```python
from build123d import *

# Parameters (mm, degrees)
SKETCH1_R                  = 13.5
BOSS_EXTRUDE1_DEPTH        = 3
CAVITY26_OUTLINE_R         = 1.85
CAVITY26_OUTLINE_R_2       = 1.7
CAVITY26_DEPTH             = 1.5
F_24_0_24_DIAMETER_HOLE1_D = 3.7
BOSS_EXTRUDE2_START        = -3
SKETCH6_R                  = 13.5
BOSS_EXTRUDE2_DEPTH        = 3
F_24_0_24_DIAMETER_HOLE2_D = 5.5
SKETCH14_W                 = 5.92
SKETCH14_H                 = 13
BOSS_EXTRUDE6_DEPTH        = 9.45
SKETCH13_R                 = 4
BOSS_EXTRUDE7_DEPTH        = 6.45
BOSS_EXTRUDE8_DEPTH        = 6.45
F_24_0_24_DIAMETER_HOLE3_D = 3.7
CUT_EXTRUDE3_DEPTH         = 9.06
SKETCH19_R                 = 2.55
CUT_EXTRUDE4_DEPTH         = 1.8
CUT_EXTRUDE5_START         = -11.2
SKETCH23_R                 = 4.233528458
CUT_EXTRUDE5_DEPTH         = 2.14
SKETCH24_W                 = 2.756109072
SKETCH24_H                 = 9.9
CUT_EXTRUDE6_DEPTH         = 10
CAVITY27_DEPTH             = 1.5
CAVITY27_START             = -6.45
CAVITY27_2_OUTLINE_R       = 3.15
CAVITY27_2_OUTLINE_R_2     = 1.85
CAVITY27_2_DEPTH           = 1.8
BOSS_EXTRUDE9_START        = 1.8
SKETCH25_R                 = 6.6
SKETCH25_R_2               = 1.85
BOSS_EXTRUDE9_DEPTH        = 1.8
SKETCH26_R                 = 4.5
CUT_EXTRUDE7_DEPTH         = 3
SKETCH27_R                 = 1.85
BOSS_EXTRUDE10_DEPTH       = 3
CUT_EXTRUDE8_START         = -1.5
CUT_EXTRUDE8_DEPTH         = 1.5
CUT_EXTRUDE9_DEPTH         = 15
F_24_0_24_DIAMETER_HOLE4_D = 3.4


# Read off the part's stored shape, not the designer's step: Cavity26, Cavity27
with BuildPart() as part:
    # Sketch1 → Boss-Extrude1 (new body)
    with BuildSketch(Plane(origin=(0, 0, 0), x_dir=(1, 0, 0), z_dir=(0, 1, 0))):
        with BuildLine():
            Line((39.88, -46.3), (44.18, -42))
            Line((44.18, -42), (44.18, 0))
            Line((44.18, 0), (7, 0))
            ThreePointArc((7, 0), (2.050252532, -2.050252532), (0, -7))
            Line((0, -7), (0, -46.3))
            Line((0, -46.3), (39.88, -46.3))
        make_face()
        with Locations(Location((23.07, -25.54, 0), (0, 0, 270))):
            Circle(SKETCH1_R, mode=Mode.SUBTRACT)
    extrude(amount=BOSS_EXTRUDE1_DEPTH)

    # Cavity26 outline → Cavity26 (cut)
    # profile 1 of 2: a face of its own
    with BuildSketch(Plane(origin=(0, 0, 0), x_dir=(1, 0, 0), z_dir=(0, 1, 0))):
        with BuildLine():
            Line((40.98, -20.5), (35.593913126, -20.5))
            ThreePointArc((35.593913126, -20.5), (36.300391291, -22.855461624), (36.567866498, -25.3))
            Line((36.567866498, -25.3), (40.93, -25.3))
            Line((40.93, -25.3), (40.93, -37.4))
            Line((40.93, -37.4), (37.464525778, -37.4))
            ThreePointArc((37.464525778, -37.4), (35.919832787, -38.039832787), (35.28, -39.584525778))
            Line((35.28, -39.584525778), (35.28, -43.05))
            Line((35.28, -43.05), (12.18, -43.05))
            Line((12.18, -43.05), (12.18, -44.675))
            Line((12.18, -44.675), (39.2422583, -44.675))
            Line((39.2422583, -44.675), (42.58, -41.3372583))
            Line((42.58, -41.3372583), (42.58, -22.55))
            Line((42.58, -22.55), (40.98, -22.55))
            Line((40.98, -22.55), (40.98, -20.5))
        make_face()
        with Locations((38.63, -40.75)):
            Circle(CAVITY26_OUTLINE_R, mode=Mode.SUBTRACT)
    # profile 2 of 2: a face of its own
    with BuildSketch(Plane(origin=(0, 0, 0), x_dir=(1, 0, 0), z_dir=(0, 1, 0))):
        with BuildLine():
            Line((40.98, -6.35), (42.58, -6.35))
            Line((42.58, -6.35), (42.58, -1.6))
            Line((42.58, -1.6), (28.18, -1.6))
            Line((28.18, -1.6), (28.18, -10.6))
            Line((28.18, -10.6), (29.56, -10.6))
            Line((29.56, -10.6), (29.56, -8.2))
            Line((29.56, -8.2), (31.16, -8.2))
            Line((31.16, -8.2), (31.16, -6.35))
            Line((31.16, -6.35), (35.06, -6.35))
            Line((35.06, -6.35), (35.06, -8.4))
            Line((35.06, -8.4), (36.21908731, -8.4))
            ThreePointArc((36.21908731, -8.4), (38.578420387, -7.150450959), (40.98, -8.31674455))
            Line((40.98, -8.31674455), (40.98, -6.35))
        make_face()
        with Locations((38.08, -3.8)):
            Circle(CAVITY26_OUTLINE_R_2, mode=Mode.SUBTRACT)
    extrude(amount=CAVITY26_DEPTH, mode=Mode.SUBTRACT)

    # Ø24.0 (24) Diameter Hole1 (through all)
    with Locations(Plane(origin=(0, 3, 0), x_dir=(1, 0, 0), z_dir=(0, 1, 0))):
        with Locations((38.63, -10.1), (38.63, -40.75), (7.73, -40.75), (7.73, -10.02)):
            Hole(F_24_0_24_DIAMETER_HOLE1_D / 2)

    # Sketch6 → Boss-Extrude2 (add)
    with BuildSketch(Plane(origin=(0, 3, 0), x_dir=(1, 0, 0), z_dir=(0, 1, 0)).offset(BOSS_EXTRUDE2_START)):
        with Locations((23.07, -25.54)):
            Circle(SKETCH6_R)
    extrude(amount=BOSS_EXTRUDE2_DEPTH)

    # Ø24.0 (24) Diameter Hole2 (through all)
    with Locations(Plane(origin=(0, 3, 0), x_dir=(1, 0, 0), z_dir=(0, 1, 0))):
        with Locations((23.07, -25.54)):
            Hole(F_24_0_24_DIAMETER_HOLE2_D / 2)

    # Sketch14 → Boss-Extrude6 (add)
    with BuildSketch(Plane(origin=(0, 3, 0), x_dir=(1, 0, 0), z_dir=(0, 1, 0))):
        with Locations((-2.96, -39.8)):
            Rectangle(SKETCH14_W, SKETCH14_H)
    extrude(amount=-BOSS_EXTRUDE6_DEPTH)

    # Sketch13 → Boss-Extrude7 (add)
    with BuildSketch(Plane(origin=(0, 0, 0), x_dir=(-1, 0, 0), z_dir=(0, -1, 0))):
        with Locations(Location((-7.73, -40.75, 0), (0, 0, 270))):
            Circle(SKETCH13_R)
    extrude(amount=BOSS_EXTRUDE7_DEPTH)

    # Sketch15 → Boss-Extrude8 (add)
    with BuildSketch(Plane(origin=(0, 0, 0), x_dir=(-1, 0, 0), z_dir=(0, -1, 0))):
        with BuildLine():
            Line((-11.002613634, -43.05), (-12.18, -43.05))
            Line((-12.18, -43.05), (-12.18, -44.675))
            Line((-12.18, -44.675), (-12.18, -46.3))
            Line((-12.18, -46.3), (0, -46.3))
            Line((0, -46.3), (0, -33.3))
            Line((0, -33.3), (-6.09, -33.3))
            Line((-6.09, -33.3), (-6.09, -37.101657911))
            ThreePointArc((-6.09, -37.101657911), (-4.371428875, -38.577443902), (-3.73, -40.75))
            ThreePointArc((-3.73, -40.75), (-6.523860401, -44.563820561), (-11.002613634, -43.05))
        make_face()
    extrude(amount=BOSS_EXTRUDE8_DEPTH)

    # Ø24.0 (24) Diameter Hole3 (through all)
    with Locations(Plane(origin=(0, 3, 0), x_dir=(1, 0, 0), z_dir=(0, 1, 0))):
        with Locations((7.73, -40.75)):
            Hole(F_24_0_24_DIAMETER_HOLE3_D / 2)

    # Sketch18 → Cut-Extrude3 (cut)
    with BuildSketch(Plane(origin=(0, 0, 33.3), x_dir=(-1, 0, 0), z_dir=(0, 0, -1))):
        Polygon((-0.43, -11.856921938), (3.17, -9.778460969), (3.17, -5.621539031), (-0.43, -3.543078062), (-4.03, -5.621539031), (-4.03, -9.778460969), align=None)
    extrude(amount=-CUT_EXTRUDE3_DEPTH, mode=Mode.SUBTRACT)

    # Sketch19 → Cut-Extrude4 (cut)
    with BuildSketch(Plane.XY.offset(46.3)):
        with Locations((0.43, -7.7)):
            Circle(SKETCH19_R)
    extrude(amount=-CUT_EXTRUDE4_DEPTH, mode=Mode.SUBTRACT)

    # Sketch23 → Cut-Extrude5 (cut)
    with BuildSketch(Plane(origin=(0, 0, 33.3), x_dir=(-1, 0, 0), z_dir=(0, 0, -1)).offset(CUT_EXTRUDE5_START)):
        with Locations((-0.43, -7.7)):
            Circle(SKETCH23_R)
    extrude(amount=CUT_EXTRUDE5_DEPTH, mode=Mode.SUBTRACT)

    # Sketch24 → Cut-Extrude6 (cut)
    with BuildSketch(Plane(origin=(0, 3, 0), x_dir=(1, 0, 0), z_dir=(0, 1, 0))):
        with Locations((-1.378054536, -39.55)):
            Rectangle(SKETCH24_W, SKETCH24_H)
    extrude(amount=-CUT_EXTRUDE6_DEPTH, mode=Mode.SUBTRACT)

    # Cavity27 outline → Cavity27 (cut)
    with BuildSketch(Plane(origin=(0, 0, 0), x_dir=(1, 0, 0), z_dir=(0, 1, 0))):
        with BuildLine():
            ThreePointArc((28.18, -21.3), (29.351572875, -24.128427125), (32.18, -25.3))
            Line((32.18, -25.3), (36.567866498, -25.3))
            ThreePointArc((36.567866498, -25.3), (36.300391291, -22.855461624), (35.593913126, -20.5))
            Line((35.593913126, -20.5), (35.06, -20.5))
            Line((35.06, -20.5), (35.06, -22.55))
            Line((35.06, -22.55), (31.16, -22.55))
            Line((31.16, -22.55), (31.16, -20.7))
            Line((31.16, -20.7), (29.56, -20.7))
            Line((29.56, -20.7), (29.56, -18.3))
            Line((29.56, -18.3), (28.18, -18.3))
            Line((28.18, -18.3), (28.18, -21.3))
        make_face()
    extrude(amount=CAVITY27_DEPTH, mode=Mode.SUBTRACT)

    # Cavity27 2 outline → Cavity27 2 (cut)
    with BuildSketch(Plane(origin=(0, 0, 0), x_dir=(1, 0, 0), z_dir=(0, 1, 0)).offset(CAVITY27_START)):
        with Locations((7.73, -40.75)):
            Circle(CAVITY27_2_OUTLINE_R)
        with Locations((7.73, -40.75)):
            Circle(CAVITY27_2_OUTLINE_R_2, mode=Mode.SUBTRACT)
    extrude(amount=CAVITY27_2_DEPTH, mode=Mode.SUBTRACT)

    # Sketch25 → Boss-Extrude9 (add)
    with BuildSketch(Plane.XZ.offset(BOSS_EXTRUDE9_START)):
        with Locations(Location((7.73, 10.02, 0), (0, 0, 90))):
            Circle(SKETCH25_R)
        with Locations(Location((7.73, 10.02, 0), (0, 0, 90))):
            Circle(SKETCH25_R_2, mode=Mode.SUBTRACT)
    extrude(amount=-BOSS_EXTRUDE9_DEPTH)

    # Sketch26 → Cut-Extrude7 (cut)
    with BuildSketch(Plane(origin=(0, -1.8, 0), x_dir=(-1, 0, 0), z_dir=(0, -1, 0))):
        with Locations(Location((-7.73, -10.02, 0), (0, 0, 90))):
            Circle(SKETCH26_R)
    extrude(amount=-CUT_EXTRUDE7_DEPTH, mode=Mode.SUBTRACT)

    # Sketch27 → Boss-Extrude10 (add)
    with BuildSketch(Plane(origin=(0, 0, 0), x_dir=(-1, 0, 0), z_dir=(0, -1, 0))):
        with Locations((-38.63, -10.1)):
            Circle(SKETCH27_R)
    extrude(amount=-BOSS_EXTRUDE10_DEPTH)

    # Sketch28 → Cut-Extrude8 (cut)
    with BuildSketch(Plane(origin=(0, 0, 0), x_dir=(-1, 0, 0), z_dir=(0, -1, 0)).offset(CUT_EXTRUDE8_START)):
        Polygon((-42.58, -22.55), (-42.58, -1.6), (-28.18, -1.6), (-28.18, -18.3), (-28.18, -43.05), (-35.28, -43.05), (-40.91112915, -43.00612915), (-42.217305027, -41.699953273), align=None)
    extrude(amount=CUT_EXTRUDE8_DEPTH, mode=Mode.SUBTRACT)

    # Sketch29 → Cut-Extrude9 (cut)
    with BuildSketch(Plane.XY.offset(46.3)):
        Polygon((0, 0), (-5.92, -5.92), (-5.92, 3), (0, 3), align=None)
    extrude(amount=-CUT_EXTRUDE9_DEPTH, mode=Mode.SUBTRACT)

    # Ø24.0 (24) Diameter Hole4 (through all)
    with Locations(Plane(origin=(0, 3, 0), x_dir=(1, 0, 0), z_dir=(0, 1, 0))):
        with Locations((38.08, -3.8)):
            Hole(F_24_0_24_DIAMETER_HOLE4_D / 2)


solid = part.part
```
Input: part model. Units: mm. Frame: model coordinates. A direction names the side the tool comes from. Give positions to 0.01 mm unless a question says otherwise; leave off trailing zeros. Order: outer loops, then holes, each group sorted by start corner. A loop starts at its lowest first (then second) coordinate and runs counter-clockwise, first axis right, second up.
1. Reachability of faces 1 (the cylindrical face through (-3.272, -5.647, 43.445)), 2 (the flat face through (2.205, -4.568, 37.767)), 3 (the flat face through (-2.756, -4, 40)), 4 (the flat face through (1, -3, 33.3)) from +Z, -Z, +X, -X, +Y, -Y: full face, straight path, thin tool, end or side. Return the list, or none.
Derived:
face 1: -Y
face 2: -Z, -Y
face 3: +Y, -Y
face 4: +X, -X, -Y
2. Pin query (flat end, axial travel): pin 1 (0.8 mm diameter, centred on y = 1, z = 21.5, fed in from -X); pin 2 (5.5 mm diameter, centred on x = 7.73, z = 40.75, fed in from -Y); pin 3 (7 mm diameter, centred on x = 7.73, z = 10.02, fed in from -Y). Return the tip coordinate at first contact, or that it passes through.
Derived:
pin 1: stops at x = 0
pin 2: stops at y = -4.65
pin 3: stops at y = 1.2
3. Section B-B on x = 23.07. Return the cut outline in (y, z) (3 decimals).
Derived:
outline: (0, 0) - (3, 0) - (3, 22.79) - (0, 22.79) - close; (0, 28.29) - (3, 28.29) - (3, 46.3) - (0, 46.3) - (0, 44.675) - (1.5, 44.675) - (1.5, 43.05) - (0, 43.05) - close
4. Material intervals for L1, parallel to X at y = 2.3, z = 40.75; L2, parallel to X at y = 2.25, z = 10.02; L3, parallel to X at y = 1.25, z = 38, sorted ascending.
Derived:
L1: x = 0 to 5.88, 9.58 to 36.78, 40.48 to 44.18
L2: x = 0 to 5.88, 9.58 to 44.18
L3: x = 0 to 28.18, 42.58 to 44.18
5. Section A-A on y = -0.75. Return the cut outline in (x, z), and give its area (3 significant figures).
Derived:
outline: (-0.75, 33.3) - (6.09, 33.3) - (6.09, 37.1) arc R4 ccw to (11, 43.05) - (12.18, 43.05) - (12.18, 46.3) - (-0.75, 46.3) - (-0.75, 44.5) - (0, 44.5) - (0, 34.6) - (-0.75, 34.6) - close; circle Ø13.2 at (7.73, 10.02); hole circle Ø9 at (7.73, 10.02); hole circle Ø3.7 at (7.73, 40.75)
area: 195 mm2
6. Section C-C on z = 40.75. Give the number of separate pieces and of enclosed holes in the cut face, and give its area (3 significant figures).
Derived:
separate pieces: 4
enclosed holes: 0
area: 140 mm2
7. Section D-D on z = 25.54. Return the cut outline in (x, y), and give its area (3 significant figures).
Derived:
outline: (0, 0) - (20.32, 0) - (20.32, 3) - (0, 3) - close; (25.82, 0) - (28.18, 0) - (28.18, 1.5) - (42.58, 1.5) - (42.58, 0) - (44.18, 0) - (44.18, 3) - (25.82, 3) - close
area: 94.4 mm2
8. Mould query, pull axis X, two halves, no side actions, for faces 5 (the flat face through (35, 1, 1.6)), 6 (the flat face through (12, -1.8, 8)), 7 (the cylindrical face through (2.1, 1.5, 2)). Classes: released by +X, released by -X, zero draft, split by the parting line, or undercut.
Derived:
face 5: undercut
face 6: zero draft
face 7: released by -X
